Read the model definition and answer for the solid it produces. Units are mm, in the model's axes. A direction names the side the tool comes from. Coordinates: 2 decimals unless noted, no trailing zeros. Order: outer loops, then holes, each group sorted by start corner. A loop starts at its lowest first (then second) coordinate and runs counter-clockwise, first axis right, second up.
```python
from build123d import *

# Parameters (mm, degrees)
SKETCH_1_W          = 35
SKETCH_1_H          = 38
EXTRUDE_1_DEPTH     = 3
SKETCH_2_R          = 0.6
CUT_EXTRUDE_1_DEPTH = 27.004807248
SKETCH_2_3_R        = 1
CUT_EXTRUDE_2_DEPTH = 1.5


with BuildPart() as part:
    # Sketch 1 → Extrude 1 (new body)
    with BuildSketch(Plane(origin=(0, 0, 0), x_dir=(1, 0, 0), z_dir=(0, 1, 0))):
        Rectangle(SKETCH_1_W, SKETCH_1_H)
    extrude(amount=EXTRUDE_1_DEPTH)

    # Sketch 2 → Cut-Extrude 1 (cut, through all)
    with BuildSketch(Plane.XZ):
        with Locations(Location((16, -11.4, 0), (0, 0, 270))):
            Circle(SKETCH_2_R)
        with Locations(Location((16, 11.4, 0), (0, 0, 270))):
            Circle(SKETCH_2_R)
        with Locations(Location((-16, 11.4, 0), (0, 0, 270))):
            Circle(SKETCH_2_R)
        with Locations(Location((-16, -11.4, 0), (0, 0, 270))):
            Circle(SKETCH_2_R)
    extrude(amount=-CUT_EXTRUDE_1_DEPTH, mode=Mode.SUBTRACT)

    # Sketch 2_3 → Cut-Extrude 2 (cut)
    with BuildSketch(Plane.XZ):
        with Locations(Location((16, -11.4, 0), (0, 0, 270))):
            Circle(SKETCH_2_3_R)
        with Locations(Location((16, 11.4, 0), (0, 0, 270))):
            Circle(SKETCH_2_3_R)
        with Locations(Location((-16, 11.4, 0), (0, 0, 270))):
            Circle(SKETCH_2_3_R)
        with Locations(Location((-16, -11.4, 0), (0, 0, 270))):
            Circle(SKETCH_2_3_R)
    extrude(amount=-CUT_EXTRUDE_2_DEPTH, mode=Mode.SUBTRACT)


solid = part.part
```
1) A cutting plane is placed at A-A, the plane z = -11.4. Determine the outline of the cut face in (x, y), and give its area (3 significant figures).
A:
outline: (-17.5, 0) - (-17, 0) - (-17, 1.5) - (-16.6, 1.5) - (-16.6, 3) - (-17.5, 3) - close; (-15.4, 1.5) - (-15, 1.5) - (-15, 0) - (15, 0) - (15, 1.5) - (15.4, 1.5) - (15.4, 3) - (-15.4, 3) - close; (16.6, 1.5) - (17, 1.5) - (17, 0) - (17.5, 0) - (17.5, 3) - (16.6, 3) - close
area: 95.4 mm2
2) Which of the six approach directions +Z, -Z, +X, -X, +Y, -Y give full straight-line access (tool end or side, diameter ignored) to faces 1 (the cylindrical face through (15.024, 0.74, -11.183)), 2 (the cylindrical face through (-15.59, 2.24, -10.96))?
A:
face 1: -Y
face 2: +Y, -Y
3) Determine the mould class of faces 3 (the cylindrical face through (16.506, 2.24, 11.077)), 4 (the flat face through (0, 0, 0)), 5 (the flat face through (-17.5, 1, 0)) for opening direction X: pulls with the +X half, pulls with the -X half, needs draft (parallel to the pull), parting line crosses it, or undercut.
A:
face 3: undercut
face 4: needs draft
face 5: pulls with the -X half
4) A flat-ended cylindrical pin translates along its axis: pin 1 Ø0.6 at (x, z) = (-16, 12) entering from -Y. Find the tip coordinate at first contact, or state that the pin passes through.
A:
pin 1: stops at y = 1.5
5) A cutting plane is placed at B-B, the plane x = -16. Determine the outline of the cut face in (y, z), and give its area (3 significant figures).
A:
outline: (0, -19) - (3, -19) - (3, -12) - (1.5, -12) - (1.5, -12.4) - (0, -12.4) - close; (0, -10.4) - (1.5, -10.4) - (1.5, -10.8) - (3, -10.8) - (3, 10.8) - (1.5, 10.8) - (1.5, 10.4) - (0, 10.4) - close; (0, 12.4) - (1.5, 12.4) - (1.5, 12) - (3, 12) - (3, 19) - (0, 19) - close
area: 104 mm2
6) Straight lines are drawn through the part: line 1 (X direction, y = 0.35, z = 11.4); line 2 (X direction, y = 2.65, z = -11.4). For each, find the intervals that lie inside material, in ascending order.
A:
line 1: x = -17.5 to -17, -15 to 15, 17 to 17.5
line 2: x = -17.5 to -16.6, -15.4 to 15.4, 16.6 to 17.5
